from build123d import *

# Parameters (mm, degrees)
ENL_V_MAT_EXTRU_1_DEPTH = 0.8


with BuildPart() as part:
    # Esquisse1 → Révolution1 (revolve)
    with BuildSketch(Plane(origin=(0, 0, 0), x_dir=(0, 0, -1), z_dir=(1, 0, 0))):
        with BuildLine():
            Line((-1.5, 0), (-1.5, 1.2))
            ThreePointArc((-1.5, 1.2), (-0.866492752, 1.926947067), (0, 2.35))
            Line((0, 2.35), (0, 1.25))
            Line((0, 1.25), (6, 1.25))
            Line((6, 1.25), (6, 0))
            Line((6, 0), (-1.5, 0))
        make_face()
    revolve(axis=Axis((0, 0, 1.5), (0, 0, 1)))

    # Esquisse2 → Enlèv. mat.-Extru.1 (cut)
    with BuildSketch(Plane.XY.offset(1.5)):
        with BuildLine():
            ThreePointArc((-0.206338407, 1.037333225), (0, 1.2), (0.206338407, 1.037333225))
            ThreePointArc((0.206338407, 1.037333225), (0.427729629, 0.74084945), (0.795187721, 0.697360915))
            ThreePointArc((0.795187721, 0.697360915), (1.039230485, 0.6), (1.001526129, 0.33997231))
            ThreePointArc((1.001526129, 0.33997231), (0.855459258, 0), (1.001526129, -0.33997231))
            ThreePointArc((1.001526129, -0.33997231), (1.039230485, -0.6), (0.795187721, -0.697360915))
            ThreePointArc((0.795187721, -0.697360915), (0.427729629, -0.74084945), (0.206338407, -1.037333225))
            ThreePointArc((0.206338407, -1.037333225), (0, -1.2), (-0.206338407, -1.037333225))
            ThreePointArc((-0.206338407, -1.037333225), (-0.427729629, -0.74084945), (-0.795187721, -0.697360915))
            ThreePointArc((-0.795187721, -0.697360915), (-1.039230485, -0.6), (-1.001526129, -0.33997231))
            ThreePointArc((-1.001526129, -0.33997231), (-0.855459258, 0), (-1.001526129, 0.33997231))
            ThreePointArc((-1.001526129, 0.33997231), (-1.039230485, 0.6), (-0.795187721, 0.697360915))
            ThreePointArc((-0.795187721, 0.697360915), (-0.427729629, 0.74084945), (-0.206338407, 1.037333225))
        make_face()
    extrude(amount=-ENL_V_MAT_EXTRU_1_DEPTH, mode=Mode.SUBTRACT)


solid = part.part
Design review of the part built by this model. Coordinates are the model's own, in mm. Round coordinates to 2 decimals unless told otherwise and drop trailing zeros. Loops run counter-clockwise (first coordinate to the right, second up) from the corner with the lowest first, then second, coordinate; pieces in that order, holes last. Notation, with made-up numbers: M 32.25,-4 L 67.25,-4 A18 cw 67.25,30 Z; hole C -11,33.5 d7. An arc over 180 degrees is marked long. Answer as a JSON object with one key per item and string values.
Item 1: We need section A-A on y = 0. Give the boundary of the cut face in (x, z).
Answer sheet:
{"outline": "M -2.35,0 L -1.25,0 L -1.25,-6 L 1.25,-6 L 1.25,0 L 2.35,0 A2.43 ccw 1.2,1.5 L 0.86,1.5 L 0.86,0.7 L -0.86,0.7 L -0.86,1.5 L -1.2,1.5 A2.43 ccw Z"}
Item 2: We need section C-C on z = -1.5. Give the boundary of the cut face in (x, y).
Answer sheet:
{"outline": "C 0,0 d2.5"}
Item 3: Clearance check with a flat-ended pin moving along its axis: P1, Ø1, axis at y = -2, z = 0.5, coming from the -X side. State where the tip first meets the part, or that it passes through.
Answer sheet:
{"P1": "stops at x = -1.64"}
Item 4: We need section B-B on x = -0.3. Give the boundary of the cut face in (y, z), and give its area (3 significant figures).
Answer sheet:
{"outline": "M -2.33,0 L -1.21,0 L -1.21,-6 L 1.21,-6 L 1.21,0 L 2.33,0 A2.41 ccw 1.16,1.5 L 0.85,1.5 L 0.85,0.7 L -0.85,0.7 L -0.85,1.5 L -1.16,1.5 A2.41 ccw Z", "area": "18.9 mm^2"}
Item 5: We need section D-D on y = 1.7. Give the boundary of the cut face in (x, z), and give its area (3 significant figures).
Answer sheet:
{"outline": "M -1.62,0 L 1.62,0 A1.73 ccw Z", "area": "2.65 mm^2"}
Item 6: The part is to be moulded in two halves that separate along Y. For faces 1 (the flat face through (1, 1, 0)), 2 (the cylindrical face through (1.22, -0.27, -3.04)), 3 (the flat face through (0, 0, 0.7)), say which applies: pulls with the +Y half, pulls with the -Y half, needs draft (parallel to the pull), parting line crosses it, or undercut.
Answer sheet:
{"face 1": "needs draft", "face 2": "parting line crosses it", "face 3": "undercut"}
Item 7: Wall thickness on L1, parallel to Z at x = 1.85, y = -0.7; L2, parallel to X at y = -1.05, z = -0.75; L3, parallel to Y at x = 0.2, z = -4.25: over which ranges is each line inside the solid? List them lowest first. Write a range as from..to.
Answer sheet:
{"L1": "z = 0..0.8", "L2": "x = -0.68..0.68", "L3": "y = -1.23..1.23"}
